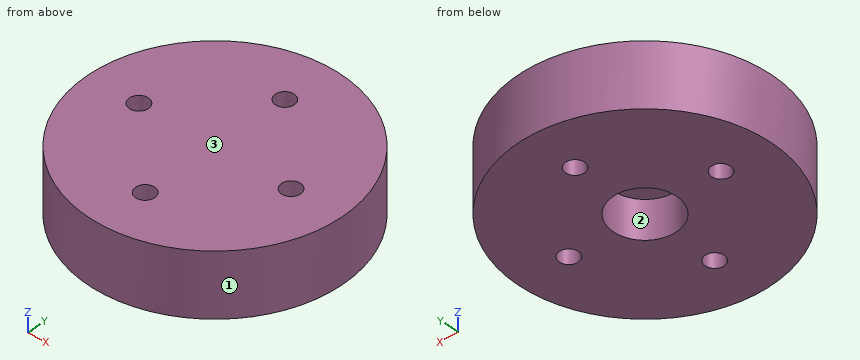
Autodesk Inventor part; units mm, degrees
ref_plane "YZ Plane" through (0, 0, 0) normal (1, 0, 0) x (0, 1, 0)
ref_plane "XZ Plane" through (0, 0, 0) normal (0, 1, 0) x (-1, 0, 0)
ref_plane "XY Plane" through (0, 0, 0) normal (0, 0, 1) x (1, 0, 0)
sketch "スケッチ1" plane through (0, 0, 0) normal (0, 0, 1) x (1, 0, 0)
  circle A0 centre (0, 0) radius 10
  dimension "d0" = 20
extrude "押し出し1" add sketch "スケッチ1" along normal blind 5
sketch "スケッチ2" plane through (0, 0, 5) normal (0, 0, 1) x (1, 0, 0)
  circle A0 centre (0, 0) radius 6
  line L0 (-6, 6) -> (6, 6)
  line L1 (6, 6) -> (6, -6)
  line L2 (6, -6) -> (-6, -6)
  line L3 (-6, -6) -> (-6, 6)
  point P0 (0, 6)
  point P1 (-6, 0)
  point P2 (0, -6)
  point P3 (6, 0)
  dimension "d3" = 12
  dimension "d6" = 360
  dimension "d8" = 6
hole "穴1" at (0, 6, 5) at (-6, 0, 5) at (0, -6, 5) at (6, 0, 5) direction (0, 0, -1) diameter 1.5 end through all
sketch "スケッチ3" plane through (0, 0, 0) normal (0, 0, -1) x (-1, 0, 0)
  circle A0 centre (0, 0) radius 2.5
  dimension "d16" = 5
extrude "押し出し2" cut sketch "スケッチ3" against normal blind 3
properties part number "servo_horn"
Geometry check sheet. Reference: the model listing, model coordinates, mm. Face numbers are marked on the shaded views. Give positions to 0.01 mm unless a question says otherwise; leave off trailing zeros. Order: outer loops, then holes, each group sorted by start corner. A loop starts at its lowest first (then second) coordinate and runs counter-clockwise, first axis right, second up. Notation, with made-up numbers: (25.25, 1) - (66.25, 1) arc R33 ccw to (66.25, 34) - close; hole circle Ø7 at (32, 17.25). An arc over 180 degrees is marked (long way). Use one line per item in the form item = value.
1) Depth check by flat-ended pin: pin 1 Ø1.5 at (y, z) = (-2.5, 1.5) entering from -X; pin 2 Ø2 at (y, z) = (3.5, 2) entering from -X. Enter the tip coordinate at first touch or a pass-through.
Working result:
pin_1 = -9.85
pin_2 = -9.68
2) Sectioned sample at C-C (y = -6). Record the boundary of the cut face in (x, z).
Working result:
outline = (-8, 0) - (-0.75, 0) - (-0.75, 5) - (-8, 5) - close; (0.75, 0) - (8, 0) - (8, 5) - (0.75, 5) - close
3) Material ranges on probe 1 along Y at (x, z) = (0, 4); probe 2 along Y at (x, z) = (0, 0.8); probe 3 along Y at (x, z) = (-5.75, 1.3), recorded low to high. Write a range as from..to.
Working result:
probe_1 = -10..-6.75, -5.25..5.25, 6.75..10
probe_2 = -10..-6.75, -5.25..-2.5, 2.5..5.25, 6.75..10
probe_3 = -8.18..-0.71, 0.71..8.18
4) Draft check along X on the marked faces 1, 2 and 3. Enter one of: released by +X, released by -X, zero draft, split by the parting line, or undercut.
Working result:
face_1 = split by the parting line
face_2 = undercut
face_3 = zero draft
5) Sectioned sample at A-A (y = 0). Record the boundary of the cut face in (x, z), and give its area (3 significant figures).
Working result:
outline = (-10, 0) - (-6.75, 0) - (-6.75, 5) - (-10, 5) - close; (-5.25, 0) - (-2.5, 0) - (-2.5, 3) - (2.5, 3) - (2.5, 0) - (5.25, 0) - (5.25, 5) - (-5.25, 5) - close; (6.75, 0) - (10, 0) - (10, 5) - (6.75, 5) - close
area = 70.0 mm^2
